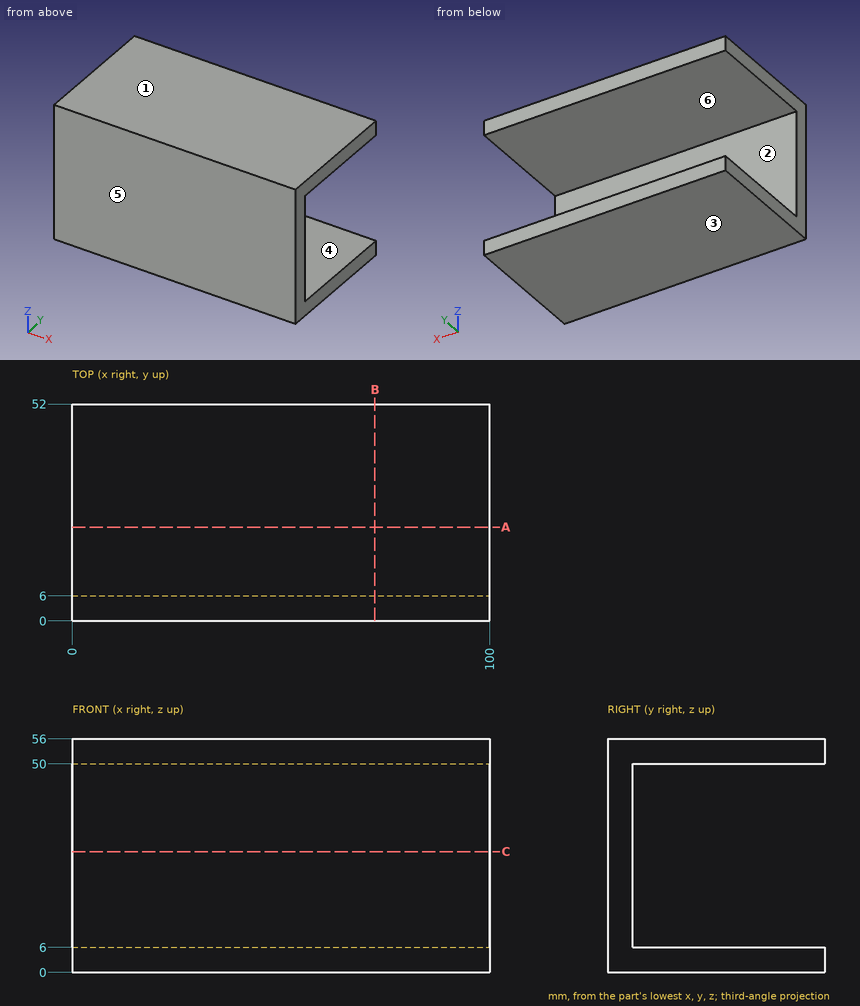
Part print with two shaded views. Sizes in mm from the minimum x, y, z corner. A direction names the side the tool comes from. Coordinates: 2 decimals unless noted, no trailing zeros. Write each loop counter-clockwise with the first axis right and the second up, starting at its lowest first coordinate (ties: lowest second). Pieces come first, ordered by that corner, then holes. Notation, with made-up numbers: (-40, 62.25) -> (9, 62.25) arc R25 cw to (9, 74.25) -> close; hole circle Ø6 at (52.5, 25.5). An arc over 180 degrees is marked (long way). Return JSON: item names as keys, results as strings. Group by question number.
Q1. Pull direction Z, two halves, no side cores. Call the marked faces 3, 4, 5 and 6: released by +Z, released by -Z, zero draft, split by the parting line, or undercut.
Q2. Drill centre lines: line 1 (Z direction, x = 42, y = 46); line 2 (Y direction, x = 62.5, z = 20.5). Where is each one in solid material? Low to high.
Q3. Cut at C-C, the plane z = 29. Give the cut face in (x, y), then the cut area to 3 significant figures.
Q4. Which spindle directions (+Z, -Z, +X, -X, +Y, -Y) get a long thin tool onto all of the face, cutting with end or side? Do the marked faces 1 and 2. Say none if no direction does.
Q5. Flat gauge pins, fed straight in: pin 1 (4 mm diameter, centred on x = 52.5, z = 37, fed in from +Y); pin 2 (5 mm diameter, centred on x = 65, y = 11, fed in from -Z). Where does each tip first touch, or does it go through?
Q6. Cut at A-A, the plane y = 22.5. Give the cut face in (x, z), then the cut area to 3 significant figures.
Q7. Cut at B-B, the plane x = 72.5. Give the cut face in (y, z).
Returned:
{
 "1": {"face 3": "released by -Z", "face 4": "undercut", "face 5": "zero draft", "face 6": "undercut"},
 "2": {"line 1": "z = 0 to 6, 50 to 56", "line 2": "y = 0 to 6"},
 "3": {"outline": "(0, 0) -> (100, 0) -> (100, 6) -> (0, 6) -> close", "area": "600 mm2"},
 "4": {"face 1": "+Z, +X, -X, +Y, -Y", "face 2": "+X, -X, +Y"},
 "5": {"pin 1": "stops at y = 6", "pin 2": "stops at z = 0"},
 "6": {"outline": "(0, 0) -> (100, 0) -> (100, 6) -> (0, 6) -> close; (0, 50) -> (100, 50) -> (100, 56) -> (0, 56) -> close", "area": "1,200 mm2"},
 "7": {"outline": "(0, 0) -> (52, 0) -> (52, 6) -> (6, 6) -> (6, 50) -> (52, 50) -> (52, 56) -> (0, 56) -> close"}
}
